Could you check a few things on this model? Use its own coordinates, in mm. Round coordinates to 2 decimals unless told otherwise and drop trailing zeros. Write each loop counter-clockwise with the first axis right and the second up, starting at its lowest first coordinate (ties: lowest second). Pieces come first, ordered by that corner, then holes. Notation, with made-up numbers: (-5, -5.75) - (7, -5.75) arc R12 cw to (7, 13.25) - close; hole circle Ø9 at (4.25, 60). An arc over 180 degrees is marked (long way). Put each result on its own line as item: value.
from build123d import *

# Parameters (mm, degrees)
SKETCH_1_R          = 21
SKETCH_1_R_2        = 15.5
EXTRUDE_1_DEPTH     = 2
CUT_EXTRUDE_START   = -2
SKETCH_3_R          = 21
CUT_EXTRUDE_1_DEPTH = 2


with BuildPart() as part:
    # 草图1 → 凸台-拉伸1 (new body)
    with BuildSketch(Plane.XY):
        Circle(SKETCH_1_R)
        Circle(SKETCH_1_R_2, mode=Mode.SUBTRACT)
    extrude(amount=EXTRUDE_1_DEPTH)

    # 草图2 → 旋转1 (revolve)
    with BuildSketch(Plane(origin=(0, 0, 0), x_dir=(1, 0, 0), z_dir=(0, 1, 0)), mode=Mode.PRIVATE) as revolve_1_sk:
        with BuildLine():
            Line((-21, 0), (-20, 0))
            ThreePointArc((-20, 0), (-18.25, 1.090097064), (-16.5, 0))
            Line((-16.5, 0), (-15.5, 0))
            ThreePointArc((-15.5, 0), (-18.25, 2.021587034), (-21, 0))
        make_face()
    revolve(revolve_1_sk.sketch.rotate(Axis((0, 0, 0), (0, 0, -1)), 180), axis=Axis((0, 0, 0), (0, 0, -1)))

    # 草图3 → 切除-拉伸1 (cut)
    with BuildSketch(Plane.XY.offset(2).offset(CUT_EXTRUDE_START)):
        Circle(SKETCH_3_R)
    extrude(amount=CUT_EXTRUDE_1_DEPTH, mode=Mode.SUBTRACT)


solid = part.part
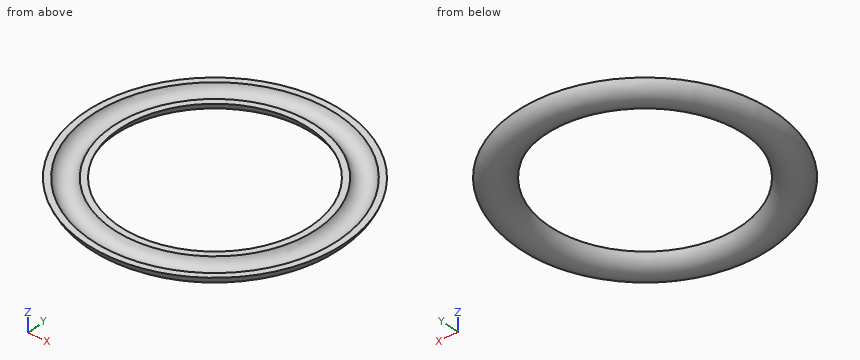
(1) Please list where these lines run through material, in increasing order: probe 1 along X at (y, z) = (-14.5, -0.5); probe 2 along Y at (x, z) = (0.5, -0.2); probe 3 along X at (y, z) = (-5.5, -0.85). Write a range as from..to.
Values found:
probe 1: x = -14.9..-13.26, -8.59..-6.05, 6.05..8.59, 13.26..14.9
probe 2: y = -20.92..-19.88, -16.61..-15.56, 15.56..16.61, 19.88..20.92
probe 3: x = -19.82..-18.38, -16.42..-14.95, 14.95..16.42, 18.38..19.82
(2) Imagine slicing it at A-A, the plane z = -0.5. List the corners of the cut face in (x, y) for me, then the cut area to 3 significant figures.
Values found:
outline: circle Ø41.58 at (0, 0); circle Ø33.71 at (0, 0); hole circle Ø39.29 at (0, 0); hole circle Ø31.42 at (0, 0)
area: 262 mm^2
(3) I'm going to push a flat-ended pin straight in: pin 1 (1 mm diameter, centred on y = 16.5, z = 0, fed in from -X). Where does the tip first touch, or does it pass through?
Values found:
pin 1: stops at x = -13.6
